For this review, take the finished solid that the model builds, in its own axes (mm). Face numbers are marked on the shaded views. A direction names the side the tool comes from. Coordinates: 2 decimals unless noted, no trailing zeros. Loops run counter-clockwise (first coordinate to the right, second up) from the corner with the lowest first, then second, coordinate; pieces in that order, holes last. Notation, with made-up numbers: (19.5, 73) -> (25.5, 73) arc R33 cw to (25.5, 106) -> close; hole circle Ø2 at (-26, -35.5). An arc over 180 degrees is marked (long way). Use a Markdown table: item, result.
from build123d import *

# Parameters (mm, degrees)
F1_DEPTH = 24
F0_R     = 8.75
F2_DEPTH = 6
F4_DEPTH = 32.5
F5_R     = 5
F6_R     = 0.75
F7_DEPTH = 6
F6_R_2   = 2.5
F8_DEPTH = 4
F0_R_2   = 8
F9_DEPTH = 5


# Not quite as in the source:
# - a pattern or mirror of a feature is missing from the dataset's text; its kind, count and spacing are read off the source's solid


with BuildPart() as f1:
    # F0 (on Top) → F1 (new body)
    with BuildSketch(Plane.XY):
        with BuildLine():
            ThreePointArc((20, -15), (-25, 0), (20, 15))
            Line((20, 15), (47.5, 15))
            Line((47.5, 15), (47.5, 27.5))
            Line((47.5, 27.5), (45.5, 27.5))
            Line((45.5, 27.5), (45.5, 21))
            Line((45.5, 21), (39.5, 21))
            Line((39.5, 21), (28, 21))
            Line((28, 21), (17.7552809046, 21))
            ThreePointArc((17.7552809046, 21), (14.2047844975, 23.5472736719), (10.295630141, 25.5))
            ThreePointArc((10.295630141, 25.5), (5.2440442409, 26.9953699734), (0, 27.5))
            ThreePointArc((0, 27.5), (-27.5, 0), (0, -27.5))
            ThreePointArc((0, -27.5), (5.2440442409, -26.9953699734), (10.295630141, -25.5))
            ThreePointArc((10.295630141, -25.5), (14.2047844975, -23.5472736719), (17.7552809046, -21))
            Line((17.7552809046, -21), (28, -21))
            Line((28, -21), (39.5, -21))
            Line((39.5, -21), (45.5, -21))
            Line((45.5, -21), (45.5, -27.5))
            Line((45.5, -27.5), (47.5, -27.5))
            Line((47.5, -27.5), (47.5, -15))
            Line((47.5, -15), (20, -15))
        make_face()
    extrude(amount=F1_DEPTH)

    # F0 (on Top) → F2 (join)
    with BuildSketch(Plane.XY):
        with BuildLine():
            Line((47.5, 15), (20, 15))
            ThreePointArc((20, 15), (-25, 0), (20, -15))
            Line((20, -15), (47.5, -15))
            Line((47.5, -15), (47.5, 15))
        make_face()
        Circle(F0_R, mode=Mode.SUBTRACT)
        with BuildLine():
            Line((45.5, 21), (45.5, 27.5))
            Line((45.5, 27.5), (0, 27.5))
            ThreePointArc((0, 27.5), (5.2440442409, 26.9953699734), (10.295630141, 25.5))
            ThreePointArc((10.295630141, 25.5), (14.2047844975, 23.5472736719), (17.7552809046, 21))
            Line((17.7552809046, 21), (28, 21))
            Line((28, 21), (39.5, 21))
            Line((39.5, 21), (45.5, 21))
        make_face()
        with BuildLine():
            Line((0, -27.5), (45.5, -27.5))
            Line((45.5, -27.5), (45.5, -21))
            Line((45.5, -21), (39.5, -21))
            Line((39.5, -21), (28, -21))
            Line((28, -21), (17.7552809046, -21))
            ThreePointArc((17.7552809046, -21), (14.2047844975, -23.5472736719), (10.295630141, -25.5))
            ThreePointArc((10.295630141, -25.5), (5.2440442409, -26.9953699734), (0, -27.5))
        make_face()
        Polygon((47.5, 27.5), (47.5, 15), (47.5, -15), (47.5, -27.5), (49.5, -27.5), (49.5, 27.5), align=None)
        with BuildLine():
            Line((45.5, 27.5), (47.5, 27.5))
            Line((47.5, 27.5), (49.5, 27.5))
            Line((49.5, 27.5), (49.5, 32.5))
            Line((49.5, 32.5), (0, 32.5))
            ThreePointArc((0, 32.5), (-32.5, 0), (0, -32.5))
            Line((0, -32.5), (49.5, -32.5))
            Line((49.5, -32.5), (49.5, -27.5))
            Line((49.5, -27.5), (47.5, -27.5))
            Line((47.5, -27.5), (45.5, -27.5))
            Line((45.5, -27.5), (0, -27.5))
            ThreePointArc((0, -27.5), (-27.5, 0), (0, 27.5))
            Line((0, 27.5), (45.5, 27.5))
        make_face()
    extrude(amount=F2_DEPTH)

    # F3 (on Front) → F4 (join, symmetric)
    with BuildSketch(Plane.XZ):
        Polygon((49.5, 6), (49.5, 0), (61.2984150648, 0), align=None)
    extrude(amount=F4_DEPTH, both=True)

    # F5
    f5_edges = [f1.edges().sort_by_distance(p)[0] for p in [
        (20, 15, 15),
        (20, -15, 15),
    ]]
    fillet(f5_edges, radius=F5_R)

    # F6 (on face) → F7 (cut, through all)
    with BuildSketch(Plane.XZ.offset(21)):
        with Locations((24, 17)):
            Circle(F6_R)
        with Locations((42.5, 17)):
            Circle(F6_R)
    f7 = extrude(amount=-F7_DEPTH, mode=Mode.SUBTRACT)

    # F7_copies: F7 across plane
    add(f7.mirror(Plane.ZX), mode=Mode.SUBTRACT)

    # F6 (on face) → F8 (cut)
    with BuildSketch(Plane.XZ.offset(21)):
        with Locations((24, 17)):
            Circle(F6_R_2)
        with Locations((24, 17)):
            Circle(F6_R, mode=Mode.SUBTRACT)
        with Locations((42.5, 17)):
            Circle(F6_R_2)
        with Locations((42.5, 17)):
            Circle(F6_R, mode=Mode.SUBTRACT)
    f8 = extrude(amount=-F8_DEPTH, mode=Mode.SUBTRACT)

    # F8_copies: F8 across plane
    add(f8.mirror(Plane.ZX), mode=Mode.SUBTRACT)

    # F0 (on Top) → F9 (join)
    with BuildSketch(Plane.XY):
        Circle(F0_R)
        Circle(F0_R_2, mode=Mode.SUBTRACT)
    extrude(amount=F9_DEPTH)


solid = f1.part
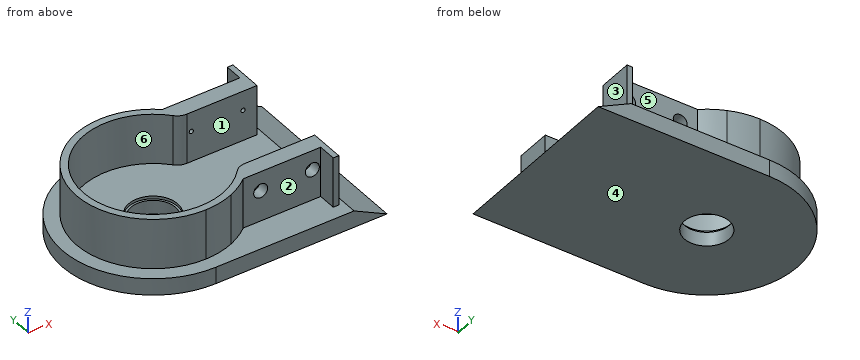
(1) Take a section at A-A on y = 0. Write out the cut boundary in (x, z).
Found:
| item | result |
|---|---|
| outline | (-32.5, 0) -> (-8, 0) -> (-8, 5) -> (-8.75, 5) -> (-8.75, 6) -> (-25, 6) -> (-25, 24) -> (-27.5, 24) -> (-27.5, 6) -> (-32.5, 6) -> close; (8, 0) -> (61.3, 0) -> (49.5, 6) -> (8.75, 6) -> (8.75, 5) -> (8, 5) -> close |
(2) Mouldability with a two-part tool opening along Y and no side actions: class the marked faces 4, 5 and 6 as pulls with the +Y half, pulls with the -Y half, needs draft (parallel to the pull), parting line crosses it, or undercut.
Found:
| item | result |
|---|---|
| face 4 | needs draft |
| face 5 | pulls with the +Y half |
| face 6 | undercut |
(3) Take a section at B-B on y = 18.5. Write out the cut boundary in (x, z), plus the area to 3 significant figures.
Found:
| item | result |
|---|---|
| outline | (-26.72, 0) -> (61.3, 0) -> (49.5, 6) -> (47.5, 6) -> (47.5, 24) -> (16.82, 24) -> (16.82, 6) -> (-16.82, 6) -> (-16.82, 24) -> (-20.35, 24) -> (-20.35, 6) -> (-26.72, 6) -> close; hole circle Ø5 at (24, 17); hole circle Ø5 at (42.5, 17) |
| area | 1,070 mm^2 |
(4) For pin 1 Ø20 at (x, y) = (0, 0) entering from +Z; pin 2 Ø1 at (y, z) = (18.5, 21.5) entering from -X; pin 3 Ø2 at (x, y) = (-8, -22) entering from -Z; pin 4 Ø12 at (y, z) = (11, 4.5) entering from -X, all flat-tipped, find the tip position at first contact; note any pin that passes through.
Found:
| item | result |
|---|---|
| pin 1 | stops at z = 6 |
| pin 2 | stops at x = -20.79 |
| pin 3 | stops at z = 0 |
| pin 4 | stops at x = -32.11 |
(5) Take a section at D-D on z = 22. Write out the cut boundary in (x, y).
Found:
| item | result |
|---|---|
| outline | (17.76, -21) -> (45.5, -21) -> (45.5, -27.5) -> (47.5, -27.5) -> (47.5, -15) -> (22.36, -15) arc R5 ccw to (18.63, -16.67) arc R25 cw (long way) to (18.63, 16.67) arc R5 ccw to (22.36, 15) -> (47.5, 15) -> (47.5, 27.5) -> (45.5, 27.5) -> (45.5, 21) -> (17.76, 21) arc R27.5 ccw (long way) to start |
(6) For the marked faces 1, 2 and 3, list the 3-axis set-ups (+Z, -Z, +X, -X, +Y, -Y) from which the entire face can be reached by the end or side of a thin tool; tool diameter is ignored.
Found:
| item | result |
|---|---|
| face 1 | +Z, +X |
| face 2 | +Z, -Y |
| face 3 | +Z, +X, +Y, -Y |
(7) For line 1 along Z through (x, y) = (24, -18); line 2 along Y through (x, z) = (0, 1.05); line 3 along Y through (x, z) = (27, 6.75), list the stretches that pass through material, from the lowest coordinate up.
Found:
| item | result |
|---|---|
| line 1 | z = 0 to 14.5, 19.5 to 24 |
| line 2 | y = -32.5 to -8, 8 to 32.5 |
| line 3 | y = -21 to -15, 15 to 21 |
(8) Take a section at C-C on x = 30. Write out the cut boundary in (y, z).
Found:
| item | result |
|---|---|
| outline | (-32.5, 0) -> (32.5, 0) -> (32.5, 6) -> (21, 6) -> (21, 24) -> (15, 24) -> (15, 6) -> (-15, 6) -> (-15, 24) -> (-21, 24) -> (-21, 6) -> (-32.5, 6) -> close |
